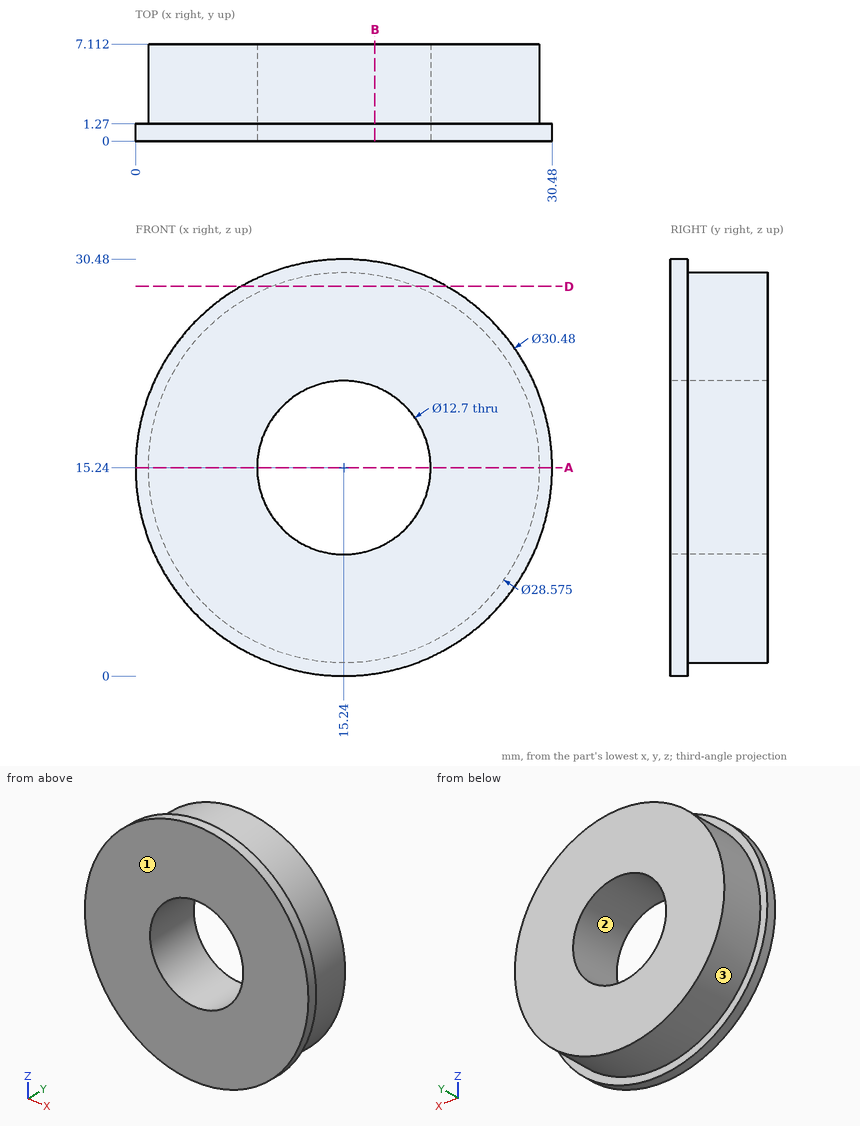
Drawing for the job (mm, zero at the part's lowest x, y, z). Round coordinates to 2 decimals unless told otherwise and drop trailing zeros. Loops run counter-clockwise (first coordinate to the right, second up) from the corner with the lowest first, then second, coordinate; pieces in that order, holes last. Notation, with made-up numbers: M -31,46.25 L 25,46.25 A29 ccw 25,83.25 Z; hole C 19.5,48.25 d7. An arc over 180 degrees is marked long. Use a Markdown table: item, result. Add a question column.
(1) Drill centre lines: line 1 (Z direction, x = 15.24, y = 2); line 2 (Z direction, x = 12, y = 5); line 3 (X direction, y = 1.75, z = 16). Where is each one in solid material? Low to high.
(2) Pull direction X, two halves, no side cores. Call the marked faces 1, 2 and 3: +X half, -X half, draft (parallel to the pull), parting line (faces both ways), or undercut.
(3) Cut at B-B (x = 17.5). Give the cut face in (y, z), and give its area (3 significant figures).
(4) Flat gauge pins, fed straight in: pin 1 (4 mm diameter, centred on y = 1, z = 27, fed in from -X); pin 2 (3 mm diameter, centred on x = 21.5, y = 6, fed in from +Z); pin 3 (6 mm diameter, centred on x = 23.5, z = 23, fed in from -Y); pin 4 (1 mm diameter, centred on x = 25.5, y = 5.5, fed in from +Z). Where does each tip first touch, or does it go through?
(5) Cut at A-A (z = 15.24). Give the cut face in (x, y), and give its area (3 significant figures).
(6) Cut at D-D (z = 28.5). Give the cut face in (x, y).
Geometry says:
| question | item | result |
|---|---|---|
| 1 | line 1 | z = 0.95 to 8.89, 21.59 to 29.53 |
| 1 | line 2 | z = 1.32 to 9.78, 20.7 to 29.16 |
| 1 | line 3 | x = 0.97 to 8.94, 21.54 to 29.51 |
| 2 | face 1 | draft |
| 2 | face 2 | undercut |
| 2 | face 3 | parting line |
| 3 | outline | M 0,0.17 L 1.27,0.17 L 1.27,1.13 L 7.11,1.13 L 7.11,9.31 L 0,9.31 Z; M 0,21.17 L 7.11,21.17 L 7.11,29.35 L 1.27,29.35 L 1.27,30.31 L 0,30.31 Z |
| 3 | area | 119 mm² |
| 4 | pin 1 | stops at x = 3.54 |
| 4 | pin 2 | stops at z = 28.71 |
| 4 | pin 3 | stops at y = 0 |
| 4 | pin 4 | stops at z = 25.67 |
| 5 | outline | M 0,0 L 8.89,0 L 8.89,7.11 L 0.95,7.11 L 0.95,1.27 L 0,1.27 Z; M 21.59,0 L 30.48,0 L 30.48,1.27 L 29.53,1.27 L 29.53,7.11 L 21.59,7.11 Z |
| 5 | area | 115 mm² |
| 6 | outline | M 7.73,0 L 22.75,0 L 22.75,1.27 L 20.56,1.27 L 20.56,7.11 L 9.92,7.11 L 9.92,1.27 L 7.73,1.27 Z |
